Study the drawing (mm; zero at the part's minimum x, y, z) and answer. Round coordinates to 2 decimals unless told otherwise and drop trailing zeros. Order: outer loops, then holes, each group sorted by start corner. A loop starts at its lowest first (then second) coordinate and runs counter-clockwise, first axis right, second up. Notation, with made-up numbers: (23, -32.5) - (39, -32.5) arc R34 cw to (39, -0.5) - close; hole circle Ø10 at (-29.5, -16). An arc over 180 degrees is marked (long way). Use one line per item in the form item = value. Start each with the question number.
Q1. The part is cut by section C-C on x = 2.5. Determine the outline of the cut face in (y, z).
Q2. For a pull along Z with two mould halves and no side action, classify the marked faces 1, 2 and 3 as +Z half, -Z half, draft (parallel to the pull), parting line (faces both ways), or undercut.
Q3. Given P1, Ø3.5, axis at x = 7.33, y = 6.35, coming from the -Z side; P2, Ø2.5, axis at x = 7.33, y = 6.35, coming from the +Z side; P3, Ø6, axis at y = 4.5, z = 29, coming from the -X side, each flat-ended and moving along its own axis, determine where each tip first touches the part or whether it passes through.
Q4. Find the intervals of material crossed by line 1 (Y direction, x = 7.5, z = 13.5) (1 decimal); line 2 (Y direction, x = 6.5, z = 11.5); line 3 (Y direction, x = 12.5, z = 19) (1 decimal), in increasing order. Write a range as [from, to].
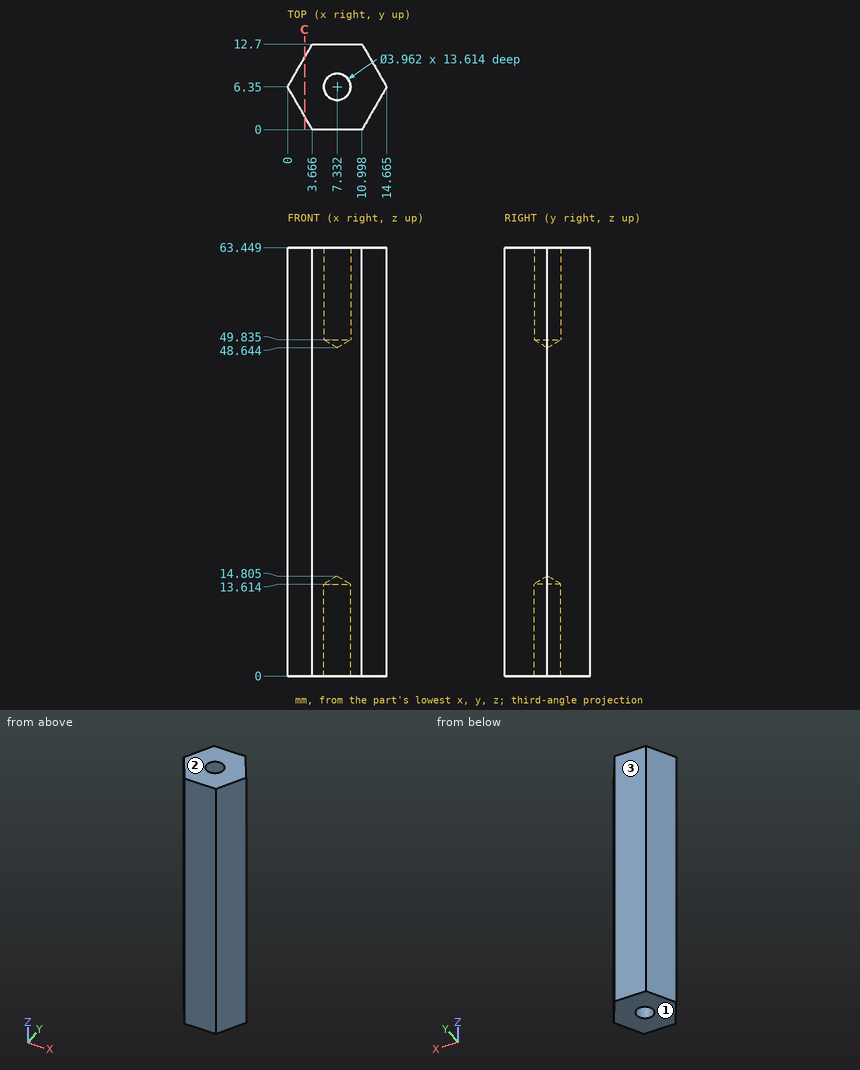
Found:
q1.outline = (2.02, 0) - (10.68, 0) - (10.68, 63.45) - (2.02, 63.45) - close
q2.face_1 = -Z half
q2.face_2 = +Z half
q2.face_3 = draft
q3.P1 = 13.75
q3.P2 = 49.4
q3.P3 = 0
q4.line_1 = [0, 4.4], [8.3, 12.7]
q4.line_2 = [0, 4.55], [8.15, 12.7]
q4.line_3 = [2.6, 10.1]
